Answer from the drawing. Dimensions are ordinates in mm from the lowest x, y and z of the part. Round coordinates to 2 decimals unless told otherwise and drop trailing zeros. Order: outer loops, then holes, each group sorted by start corner. A loop starts at its lowest first (then second) coordinate and runs counter-clockwise, first axis right, second up.
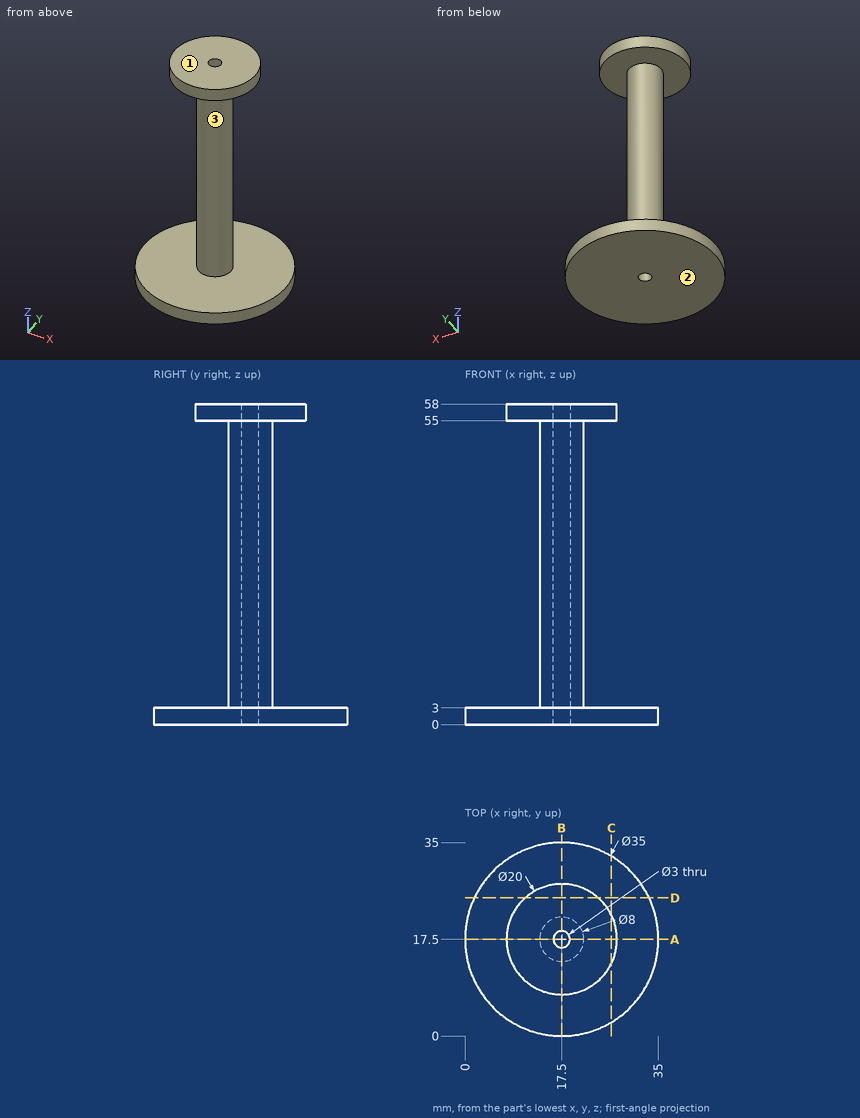
Q1. Straight lines are drawn through the part: probe 1 along Z at (x, y) = (19, 11.5); probe 2 along Y at (x, z) = (17.5, 21.5); probe 3 along Z at (x, y) = (16.5, 30). For each, find the intervals that lie inside material, in ascending order.
Outcome:
probe 1: z = 0 to 3, 55 to 58
probe 2: y = 13.5 to 16, 19 to 21.5
probe 3: z = 0 to 3
Q2. A cutting plane is placed at A-A, the plane y = 17.5. Give the vertices of the cut face in (x, z), plus the area to 3 significant figures.
Outcome:
outline: (0, 0) - (16, 0) - (16, 58) - (7.5, 58) - (7.5, 55) - (13.5, 55) - (13.5, 3) - (0, 3) - close; (19, 0) - (35, 0) - (35, 3) - (21.5, 3) - (21.5, 55) - (27.5, 55) - (27.5, 58) - (19, 58) - close
area: 407 mm2
Q3. Flat-ended cylindrical pins translate along their axes: pin 1 (12 mm diameter, centred on y = 15.5, z = 48.5, fed in from +X); pin 2 (5 mm diameter, centred on x = 9.5, y = 30, fed in from -Z); pin 3 (6 mm diameter, centred on y = 11, z = 44, fed in from -X); pin 4 (8 mm diameter, centred on x = 4.5, z = 6.5, fed in from +Y). Find the tip coordinate at first contact, or state that the pin passes through.
Outcome:
pin 1: stops at x = 21.5
pin 2: stops at z = 0
pin 3: stops at x = 15.56
pin 4: stops at y = 31.06
Q4. A cutting plane is placed at D-D, the plane y = 25. Give the vertices of the cut face in (x, z), plus the area to 3 significant figures.
Outcome:
outline: (1.69, 0) - (33.31, 0) - (33.31, 3) - (1.69, 3) - close; (10.89, 55) - (24.11, 55) - (24.11, 58) - (10.89, 58) - close
area: 135 mm2
Q5. A cutting plane is placed at C-C, the plane x = 26.5. Give the vertices of the cut face in (y, z), plus the area to 3 significant figures.
Outcome:
outline: (2.49, 0) - (32.51, 0) - (32.51, 3) - (2.49, 3) - close; (13.14, 55) - (21.86, 55) - (21.86, 58) - (13.14, 58) - close
area: 116 mm2
Q6. For a pull along Z with two mould halves and no side action, classify the marked faces 1, 2 and 3 as released by +Z, released by -Z, zero draft, split by the parting line, or undercut.
Outcome:
face 1: released by +Z
face 2: released by -Z
face 3: undercut
